For this review, take the finished solid that the model builds, in its own axes (mm). A direction names the side the tool comes from. Coordinates: 2 decimals unless noted, no trailing zeros. Loops run counter-clockwise (first coordinate to the right, second up) from the corner with the lowest first, then second, coordinate; pieces in that order, holes last. Notation, with made-up numbers: M -40,50 L -17,50 A8 ccw -17,58 Z; hole C 73,-6.75 d9. An arc over 180 degrees is marked long. Put each result on its own line as item: value.
```python
from build123d import *

# Parameters (mm, degrees)
F0_R        = 67
F0_R_2      = 59.6
F1_DEPTH    = 3.75
F2_R        = 63.875
F2_R_2      = 63.125
F3_DEPTH    = 1.5
F3_FACE_R   = 67
F3_FACE_R_2 = 63.875
F4_DEPTH    = 2


with BuildPart() as f1:
    # F0 (on Front) → F1 (new body, symmetric)
    with BuildSketch(Plane.XZ):
        Circle(F0_R)
        Circle(F0_R_2, mode=Mode.SUBTRACT)
    extrude(amount=F1_DEPTH, both=True)

    # F2 (on face) → F3 (cut)
    with BuildSketch(Plane.XZ.offset(3.75)):
        Circle(F2_R)
        Circle(F2_R_2, mode=Mode.SUBTRACT)
    extrude(amount=-F3_DEPTH, mode=Mode.SUBTRACT)

    # F3_face (on face) → F4 (cut)
    with BuildSketch(Plane.XZ.offset(3.75)):
        Circle(F3_FACE_R)
        Circle(F3_FACE_R_2, mode=Mode.SUBTRACT)
    extrude(amount=-F4_DEPTH, mode=Mode.SUBTRACT)


solid = f1.part
```
(1) Add section B-B (z = -11.5). Write out the cut boundary in (x, y).
Determined:
outline: M -66.01,-1.75 L -62.83,-1.75 L -62.83,-2.25 L -62.07,-2.25 L -62.07,-3.75 L -58.48,-3.75 L -58.48,3.75 L -66.01,3.75 Z; M 58.48,-3.75 L 62.07,-3.75 L 62.07,-2.25 L 62.83,-2.25 L 62.83,-1.75 L 66.01,-1.75 L 66.01,3.75 L 58.48,3.75 Z
(2) For pin 1 (2 mm diameter, centred on y = 0.5, z = 40, fed in from +X); pin 2 (3 mm diameter, centred on x = 16, y = 2.5, fed in from -Z); pin 3 (1 mm diameter, centred on y = -2.5, z = 10, fed in from +X), all flat-tipped, find the tip position at first contact; note any pin that passes through.
Determined:
pin 1: stops at x = 54.48
pin 2: stops at z = -65.41
pin 3: stops at x = 63.15
(3) Wall thickness on line 1 along Z through (x, y) = (0, 1.5); line 2 along Z through (x, y) = (-50, 3.25); line 3 along X through (y, z) = (-1, 34.5): over which ranges is each line inside the solid? List them lowest first. Write a range as [from, to].
Determined:
line 1: z = [-67, -59.6], [59.6, 67]
line 2: z = [-44.6, -32.44], [32.44, 44.6]
line 3: x = [-57.43, -48.6], [48.6, 57.43]
(4) Draft analysis for pull direction Z (two halves, no side actions). For faces 3 (the cylindrical face through (56.85, 0.05, 17.9)), 4 (the cylindrical face through (-13.847, -2.003, -62.356)), 5 (the flat face through (-62, -2.25, 14)), state which applies: +Z half, -Z half, draft (parallel to the pull), parting line (faces both ways), or undercut.
Determined:
face 3: undercut
face 4: parting line
face 5: draft
(5) Add section A-A (x = 0). Write out the cut boundary in (y, z) (3 decimals), plus the area to 4 significant figures.
Determined:
outline: M -3.75,-63.125 L -2.25,-63.125 L -2.25,-63.875 L -1.75,-63.875 L -1.75,-67 L 3.75,-67 L 3.75,-59.6 L -3.75,-59.6 Z; M -3.75,59.6 L 3.75,59.6 L 3.75,67 L -1.75,67 L -1.75,63.875 L -2.25,63.875 L -2.25,63.125 L -3.75,63.125 Z
area: 96.25 mm^2
(6) Tool access review of faces 1 (the cylindrical face through (-8.218, -3.01, 62.588)), 2 (the flat face through (-45, 3.75, -39.4)): name each direction out of +Z, -Z, +X, -X, +Y, -Y from which nothing blocks a thin tool from reaching the whole face with its end or side.
Determined:
face 1: -Y
face 2: +Z, -Z, +X, -X, +Y
